Source: three-view drawing plus pictorial views. Frame: mm from the lowest corner of the part. A direction names the side the tool comes from. Coordinates: 2 decimals unless noted, no trailing zeros. Write each loop counter-clockwise with the first axis right and the second up, starting at its lowest first coordinate (ties: lowest second). Pieces come first, ordered by that corner, then holes. Notation, with made-up numbers: M -24.5,-14 L -8.5,-14 A17 ccw -8.5,1 Z; hole C 59.25,81 d6. An arc over 180 degrees is marked long. Write item = value, one per line. Start each with the question number.
Item 1: Section A-A on y = 10.25. Output: boundary loops of the cut face in (x, z) (3 decimals), plus the area to 3 significant figures.
Item 2: Ray query, L1, parallel to Y at x = 10.25, z = 8.75; L2, parallel to Z at x = 17.25, y = 7; L3, parallel to Y at x = 10.25, z = 14.75 (3 decimals). Return the intervals inside material, ascending. Write a range as [from, to].
Item 3: Section C-C on z = 14.25. Output: boundary loops of the cut face in (x, y) (3 decimals), plus the area to 3 significant figures.
Item 4: Reachability of the marked faces 1, 2 and 3 from +Z, -Z, +X, -X, +Y, -Y: full face, straight path, thin tool, end or side. Return the list, or none.
Item 5: First-contact query: pin 1 Ø9 at (x, y) = (10.25, 10.25) entering from -Z; pin 2 Ø8 at (y, z) = (4, 7) entering from -X; pin 3 Ø8 at (y, z) = (17, 6.5) entering from -X; pin 4 Ø3 at (x, y) = (9.5, 9.5) entering from -Z. Flat tips, straight axial feed; report the tip coordinate or a pass-through.
Item 6: Pull-direction query (X, two-part tool) for the marked faces 4, 5, 6 and 7; classes: +X half, -X half, draft (parallel to the pull), parting line (faces both ways), or undercut.
Item 7: Section D-D on y = 18.25. Output: boundary loops of the cut face in (x, z).
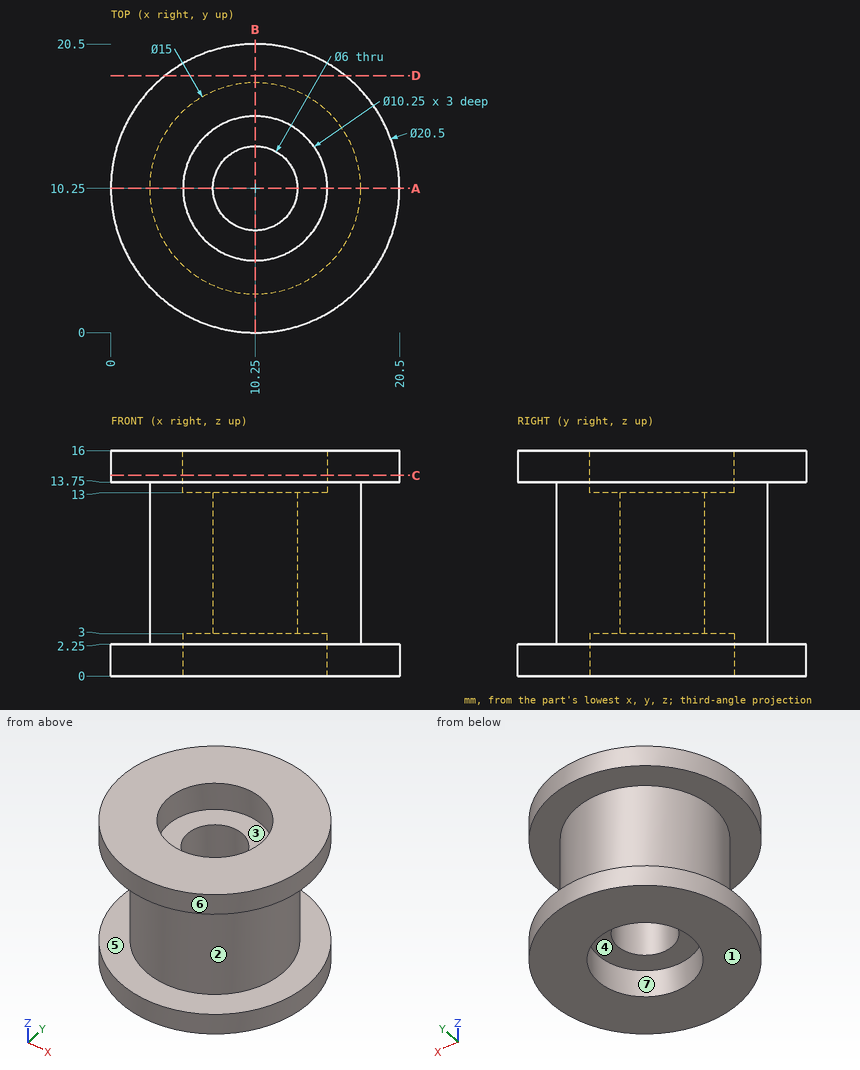
Responses:
q1.outline = M 0,0 L 5.125,0 L 5.125,3 L 7.25,3 L 7.25,13 L 5.125,13 L 5.125,16 L 0,16 L 0,13.75 L 2.75,13.75 L 2.75,2.25 L 0,2.25 Z; M 13.25,3 L 15.375,3 L 15.375,0 L 20.5,0 L 20.5,2.25 L 17.75,2.25 L 17.75,13.75 L 20.5,13.75 L 20.5,16 L 15.375,16 L 15.375,13 L 13.25,13 Z
q1.area = 143 mm²
q2.L1 = [2.75, 7.25], [13.25, 17.75]
q2.L2 = [0, 2.25], [13.75, 16]
q2.L3 = [0, 5.125], [15.375, 20.5]
q3.outline = C 10.25,10.25 d20.5; hole C 10.25,10.25 d10.25
q3.area = 248 mm²
q4.face_1 = -Z, +X, -X, +Y, -Y
q4.face_2 = none
q4.face_3 = +Z
q5.pin_1 = 3
q5.pin_2 = 3.1
q5.pin_3 = 3.27
q5.pin_4 = through
q6.face_4 = undercut
q6.face_5 = draft
q6.face_6 = parting line
q6.face_7 = undercut
q7.outline = M 3.84,0 L 16.66,0 L 16.66,2.25 L 3.84,2.25 Z; M 3.84,13.75 L 16.66,13.75 L 16.66,16 L 3.84,16 Z
